Answer from the drawing. Dimensions are ordinates in mm from the lowest x, y and z of the part. Round coordinates to 2 decimals unless told otherwise and drop trailing zeros. Write each loop counter-clockwise with the first axis right and the second up, starting at its lowest first coordinate (ties: lowest second). Pieces come first, ordered by that corner, then holes. Notation, with made-up numbers: (13.25, 13.25) - (69.25, 13.25) arc R19 ccw to (69.25, 50.25) - close; hole circle Ø5 at (24, 57.25). An arc over 180 degrees is marked (long way). Return JSON: item names as keys, results as strings. Group by question number.
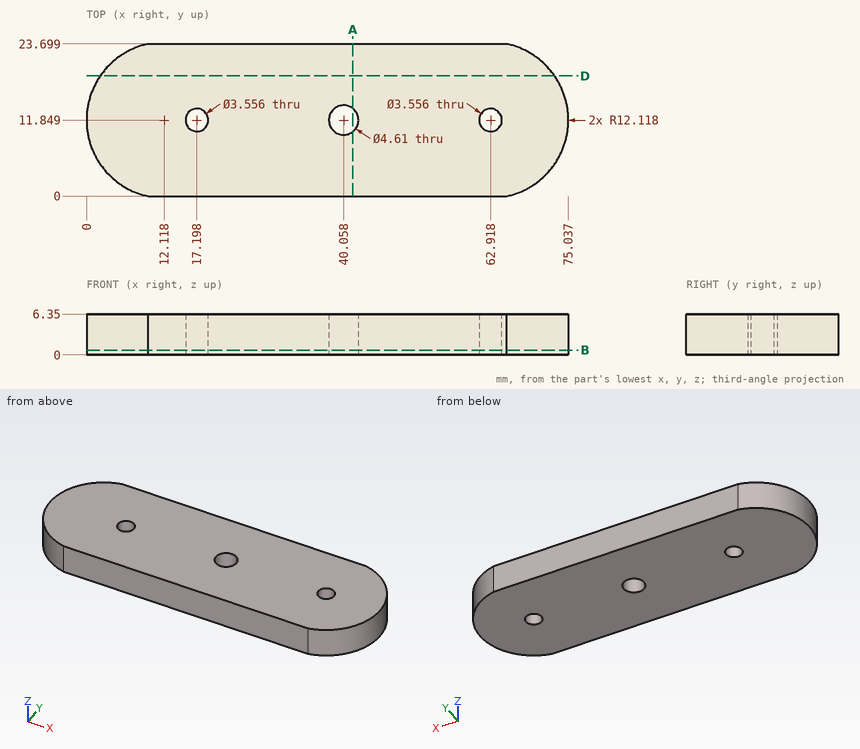
(1) Find section B-B (z = 0.75). State how many separate pieces and enclosed holes the cut face has, plus the area to 3 significant figures.
(2) Flat-ended cylindrical pins translate along their axes: pin 1 (10 mm diameter, centred on x = 40, y = 14, fed in from -Z); pin 2 (3 mm diameter, centred on x = 62.92, y = 11.85, fed in from -Z). Find the tip coordinate at first contact, or state that the pin passes through.
(3) Find section D-D (y = 18.75). Write down the section's boundary in (x, z), plus the area to 3 significant figures.
(4) Find section A-A (x = 41.5). Write down the section's boundary in (y, z).
(5) Consider line 1 (Y direction, x = 41, z = 6) (1 decimal); line 2 (X direction, y = 10, z = 4.5) (1 decimal); line 3 (Y direction, x = 63.5, z = 3.75). Determine where each line is inside the solid, lowest interval first.
Check sheet entries:
{
 "1": {"separate pieces": "1", "enclosed holes": "3", "area": "1,630 mm^2"},
 "2": {"pin 1": "stops at z = 0", "pin 2": "passes through"},
 "3": {"outline": "(2.16, 0) - (72.88, 0) - (72.88, 6.35) - (2.16, 6.35) - close", "area": "449 mm^2"},
 "4": {"outline": "(0, 0) - (10.05, 0) - (10.05, 6.35) - (0, 6.35) - close; (13.65, 0) - (23.7, 0) - (23.7, 6.35) - (13.65, 6.35) - close"},
 "5": {"line 1": "y = 0 to 9.7, 14 to 23.7", "line 2": "x = 0.1 to 38.7, 41.4 to 74.9", "line 3": "y = 0 to 10.17, 13.53 to 23.7"}
}
